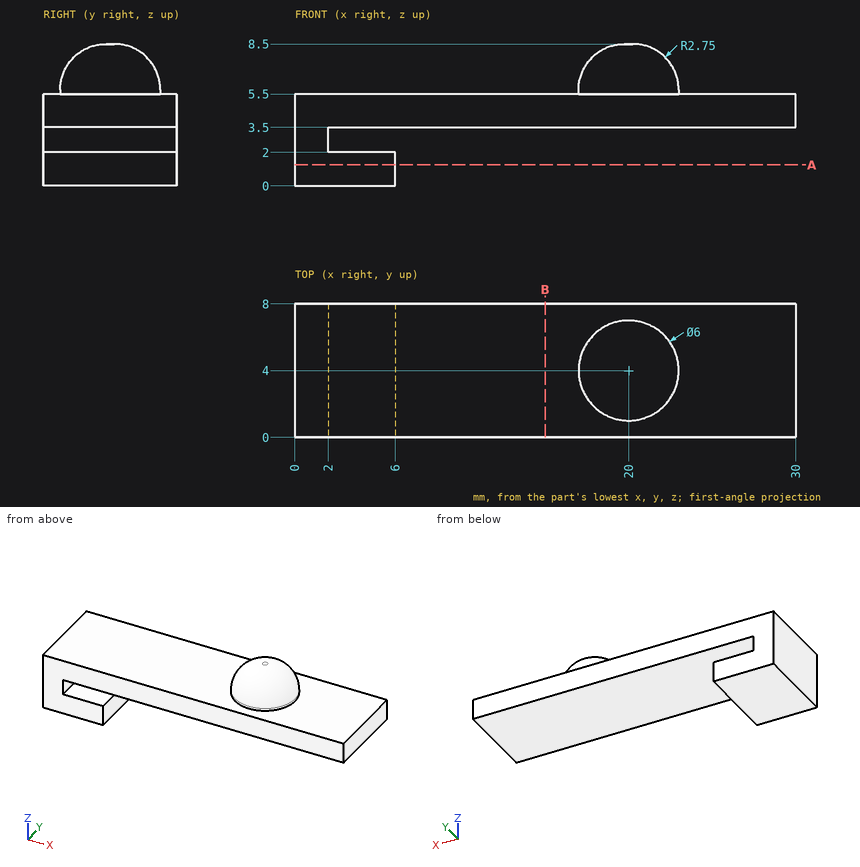
Can you work these out from the drawing? Everything is in mm from the part's minimum corner. Round coordinates to 2 decimals unless told otherwise and drop trailing zeros. Loops run counter-clockwise (first coordinate to the right, second up) from the corner with the lowest first, then second, coordinate; pieces in that order, holes last. Notation, with made-up numbers: (89, 82.5) - (97, 82.5) arc R36 cw to (97, 118.5) - close; hole circle Ø4 at (51.25, 38). An arc over 180 degrees is marked (long way). Answer in a Markdown table with one row per item. Add a question column.
(1) If we section it at B-B (x = 15): Please give me the cut outline in (y, z).
(2) I'm going to push flat-ended pins straight in: pin 1 (0.6 mm diameter, centred on y = 3, z = 1, fed in from +X); pin 2 (5 mm diameter, centred on x = 20.5, z = 6, fed in from -Y); pin 3 (0.8 mm diameter, centred on y = 6, z = 2.5, fed in from +X); pin 4 (3 mm diameter, centred on x = 15, y = 3.5, fed in from +Z). Where does each tip first touch, or does it pass through?
(3) I need wall thicknesses on line 1 along Z through (x, y) = (3.5, 7); line 2 along Z through (x, y) = (14.25, 7); line 3 along X through (y, z) = (7.5, 1.75). Which ranges of each line are inside material? Lowest first, please.
(4) If we section it at A-A (z = 1.25): Please give me the cut outline in (x, y), plus the area to 3 significant figures.
Model answer:
| question | item | result |
|---|---|---|
| 1 | outline | (0, 3.5) - (8, 3.5) - (8, 5.5) - (0, 5.5) - close |
| 2 | pin 1 | stops at x = 6 |
| 2 | pin 2 | stops at y = 0 |
| 2 | pin 3 | stops at x = 2 |
| 2 | pin 4 | stops at z = 5.5 |
| 3 | line 1 | z = 0 to 2, 3.5 to 5.5 |
| 3 | line 2 | z = 3.5 to 5.5 |
| 3 | line 3 | x = 0 to 6 |
| 4 | outline | (0, 0) - (6, 0) - (6, 8) - (0, 8) - close |
| 4 | area | 48.0 mm² |
